```python
from build123d import *

# Parameters (mm, degrees)
EXTRUDE_1_DEPTH     = 3
SKETCH_2_R          = 5.5
CUT_EXTRUDE_1_DEPTH = 38.72513216


with BuildPart() as part:
    # Эскиз1 → Бобышка-Вытянуть1 (new body)
    with BuildSketch(Plane(origin=(0, 0, 0), x_dir=(0, 0, -1), z_dir=(1, 0, 0))):
        Polygon((9.642962643, 36.348299382), (-9.642962643, 36.348299382), (-9.642962643, -18.220164561), (4.520288528, -36.348299382), (9.642962643, -36.348299382), align=None)
    extrude(amount=EXTRUDE_1_DEPTH)

    # Эскиз2 → Вырез-Вытянуть1 (cut, through all)
    with BuildSketch(Plane.ZY):
        with Locations((0, 16.706183396)):
            Circle(SKETCH_2_R)
    extrude(amount=-CUT_EXTRUDE_1_DEPTH, mode=Mode.SUBTRACT)


solid = part.part
```
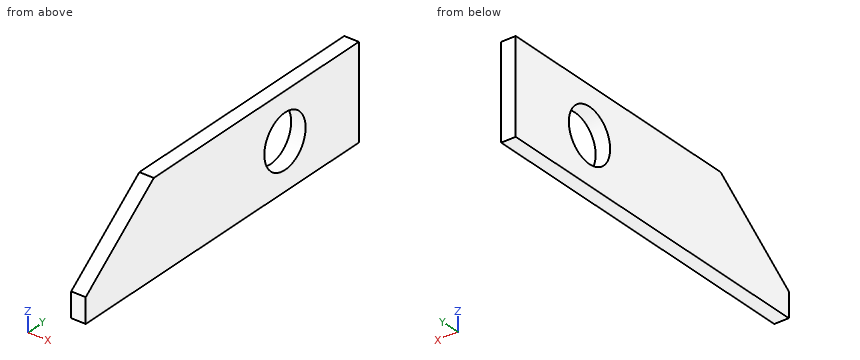
Part model, mm, in its own coordinate system. Round coordinates to 2 decimals unless told otherwise and drop trailing zeros. Loops run counter-clockwise (first coordinate to the right, second up) from the corner with the lowest first, then second, coordinate; pieces in that order, holes last. Notation, with made-up numbers: (-6.75, 0.5) -> (43.25, 0.5) arc R26 cw to (43.25, 35.5) -> close; hole circle Ø2 at (87, 79.5). An arc over 180 degrees is marked (long way). Use one line per item in the form item = value. Start each with the question number.
Item 1: Drill centre lines: line 1 along Y through (x, z) = (2.1, 0); line 2 along Y through (x, z) = (0.95, -3.5); line 3 along Z through (x, y) = (2.5, 14.5). Where is each one in solid material? Low to high.
Item 2: Band-saw the part on C-C (x = 0.8). List the corners of the cut face in (y, z), plus the area to 3 significant figures.
Item 3: Band-saw the part on D-D (z = 7.5). List the corners of the cut face in (x, y), plus the area to 3 significant figures.
Item 4: Band-saw the part on B-B (y = 21). List the corners of the cut face in (x, z).
Item 5: Drop a flat-ended pin along its axis: pin 1 Ø1.5 at (x, z) = (2, 1.5) entering from -Y. Give the stop position or say it passes through.
Item 6: Band-saw the part on A-A (z = 4). List the corners of the cut face in (x, y).
Data:
q1.line_1 = -30.56 to 11.21, 22.21 to 36.35
q1.line_2 = -35.04 to 12.46, 20.95 to 36.35
q1.line_3 = -9.64 to -5.04, 5.04 to 9.64
q2.outline = (-36.35, -9.64) -> (36.35, -9.64) -> (36.35, 9.64) -> (-18.22, 9.64) -> (-36.35, -4.52) -> close; hole circle Ø11 at (16.71, 0)
q2.area = 1,180 mm^2
q3.outline = (0, -20.96) -> (3, -20.96) -> (3, 36.35) -> (0, 36.35) -> close
q3.area = 172 mm^2
q4.outline = (0, -9.64) -> (3, -9.64) -> (3, -3.44) -> (0, -3.44) -> close; (0, 3.44) -> (3, 3.44) -> (3, 9.64) -> (0, 9.64) -> close
q5.pin_1 = -29.6
q6.outline = (0, -25.44) -> (3, -25.44) -> (3, 12.93) -> (0, 12.93) -> close; (0, 20.48) -> (3, 20.48) -> (3, 36.35) -> (0, 36.35) -> close
